Part model, mm, in its own coordinate system. A direction names the side the tool comes from. Give positions to 0.01 mm unless a question says otherwise; leave off trailing zeros. Order: outer loops, then holes, each group sorted by start corner. A loop starts at its lowest first (then second) coordinate and runs counter-clockwise, first axis right, second up. Notation, with made-up numbers: (66.5, 55.25) -> (112.5, 55.25) arc R23 cw to (112.5, 67.25) -> close; hole circle Ø6 at (49, -20). An arc over 180 degrees is marked (long way). Write item = value, one per line. Start each with the question number.
(1) Saw through at A-A, the plane y = -16.5. List the corners of the cut face in (x, z).
(2) Which spindle directions (+Z, -Z, +X, -X, +Y, -Y) get a long thin tool onto all of the face, cutting with end or side? Do faces 1 (the flat face through (5.988, -10.977, 4.93)), 2 (the flat face through (-30, 0, 5)). Say none if no direction does.
(3) Saw through at B-B, the plane z = 5.75. List the corners of the cut face in (x, y).
(4) Probe line 1 along X through (y, z) = (-9.5, 0.5); line 2 along X through (y, z) = (-19.5, 3.75) (3 decimals); line 3 along Y through (x, z) = (15, 2.75). List the from-to ranges inside material, lowest first. Write a range as from..to.
(5) Saw through at C-C, the plane x = 14. List the corners of the cut face in (y, z).
(6) Two-plate mould, pull along X, no slides. Class faces 3 (the flat face through (6.512, 10.674, 4.93)), 4 (the flat face through (0, -30, 5)), 5 (the flat face through (30, 0, 5)): pulls with the +X half, pulls with the -X half, needs draft (parallel to the pull), parting line crosses it, or undercut.
from build123d import *

# Parameters (mm, degrees)
SCHIZZO1_W                   = 60
SCHIZZO1_H                   = 60
ESTRUSIONE_ESTRUSIONE1_DEPTH = 10


with BuildPart() as part:
    # Schizzo1 → Estrusione-Estrusione1 (new body)
    with BuildSketch(Plane.XY):
        Rectangle(SCHIZZO1_W, SCHIZZO1_H)
        Polygon((25, 0), (-12.5, 21.650635095), (-12.5, -21.650635095), align=None, mode=Mode.SUBTRACT)
    extrude(amount=ESTRUSIONE_ESTRUSIONE1_DEPTH)


solid = part.part
Results list:
q1.outline = (-30, 0) -> (-12.5, 0) -> (-12.5, 10) -> (-30, 10) -> close; (-3.58, 0) -> (30, 0) -> (30, 10) -> (-3.58, 10) -> close
q2.face_1 = +Z, -Z
q2.face_2 = +Z, -Z, -X, +Y, -Y
q3.outline = (-30, -30) -> (30, -30) -> (30, 30) -> (-30, 30) -> close; hole (-12.5, -21.65) -> (25, 0) -> (-12.5, 21.65) -> close
q4.line_1 = -30..-12.5, 8.55..30
q4.line_2 = -30..-12.5, -8.775..30
q4.line_3 = -30..-5.77, 5.77..30
q5.outline = (-30, 0) -> (-6.35, 0) -> (-6.35, 10) -> (-30, 10) -> close; (6.35, 0) -> (30, 0) -> (30, 10) -> (6.35, 10) -> close
q6.face_3 = undercut
q6.face_4 = needs draft
q6.face_5 = pulls with the +X half
